Can you work these out from the model? Positions are in its coordinate system, mm. Face numbers are marked on the shaded views. A direction names the side the tool comes from. Give positions to 0.01 mm unless a question says otherwise; leave off trailing zeros. Write each loop counter-clockwise with the first axis right and the second up, starting at its lowest first coordinate (ties: lowest second). Pieces come first, ordered by that corner, then holes.
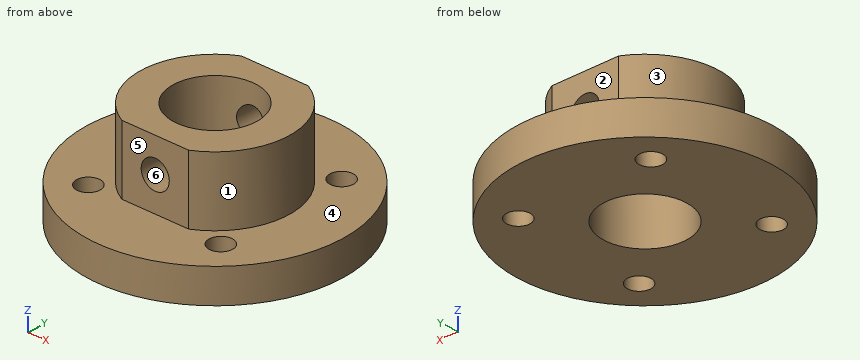
Autodesk Inventor part; units mm, degrees
ref_plane "YZ Plane" through (0, 0, 0) normal (1, 0, 0) x (0, 1, 0)
ref_plane "XZ Plane" through (0, 0, 0) normal (0, 1, 0) x (-1, 0, 0)
ref_plane "XY Plane" through (0, 0, 0) normal (0, 0, 1) x (1, 0, 0)
sketch "スケッチ1" plane through (0, 0, 0) normal (0, 0, 1) x (1, 0, 0)
  circle A0 centre (0, 0) radius 19
  circle A1 centre (0, 0) radius 14
  circle A2 centre (-14, 0) radius 1.75
  circle A3 centre (0, -14) radius 1.75
  circle A4 centre (14, 0) radius 1.75
  circle A5 centre (0, 14) radius 1.75
  line L0 (-19, 0) -> (19, 0)
  dimension "d10" = 28
  dimension "d0" = 38
  dimension "d11" = 3.5
  dimension "d14" = 360
extrude "押し出し1" add sketch "スケッチ1" along normal blind 5
sketch "スケッチ2" plane through (0, 0, 5) normal (0, 0, 1) x (1, 0, 0)
  circle A0 centre (0, 0) radius 11
  line L0 (5, -9.798) -> (-5, -9.798)
  line L1 (-5, -9.798) -> (-5, 9.798)
  line L2 (-5, 9.798) -> (5, 9.798)
  line L3 (5, 9.798) -> (5, -9.798)
  line L4 (5, -9.798) -> (-5, 9.798) construction
  line L5 (-5, -9.798) -> (5, 9.798) construction
  dimension "d3" = 22
  dimension "d6" = 10
extrude "押し出し2" add sketch "スケッチ2" along normal blind 10 contours A0 L3 | L3 L0 L1 L2 | L1 A0
sketch "スケッチ3" plane through (0, 0, 0) normal (0, 0, -1) x (-1, 0, 0)
  circle A0 centre (0, 0) radius 6.2
  dimension "d7" = 12.4
extrude "押し出し3" cut sketch "スケッチ3" against normal blind 30
sketch "スケッチ4" plane through (0, 0, 0) normal (0, 0, -1) x (-1, 0, 0)
  circle A0 centre (0, 0) radius 14
  point P0 (-14, 0)
  point P1 (-9.8995, -9.8995)
  point P2 (0, -14)
  point P3 (9.8995, -9.8995)
  point P4 (14, 0)
  point P5 (9.8995, 9.8995)
  point P6 (0, 14)
  point P7 (-9.8995, 9.8995)
  dimension "d16" = 28
  dimension "d33" = 360
hole "穴1" at (9.8995, -9.8995, 0) at (9.8995, 9.8995, 0) at (-9.8995, 9.8995, 0) at (-9.8995, -9.8995, 0) direction (0, 0, 1) diameter 3.5 end through all
sketch "スケッチ5" plane through (-5, 9.798, 5) normal (0, 1, 0) x (1, 0, 0)
  line L0 (10, -10) -> (0, -10)
  line L1 (5, -10) -> (5, 0)
  line L2 (0, 0) -> (10, 0)
  point P0 (5, 5)
  point P1 (5, -5)
hole "穴2" at (0, 9.798, 10) direction (0, -1, 0) diameter 4.2 end through all
properties part number "light_tire_fixer_10"
(1) Imagine slicing it at B-B, the plane y = 0. Write out the boundary of the cut face in (x, z).
Returned:
outline: (-19, 0) - (-6.2, 0) - (-6.2, 15) - (-11, 15) - (-11, 5) - (-19, 5) - close; (6.2, 0) - (19, 0) - (19, 5) - (11, 5) - (11, 15) - (6.2, 15) - close
(2) If I drill on L1, parallel to Z at x = 0, y = -8; L2, parallel to X at y = 9, z = 3.75; L3, parallel to X at y = 10.5, z = 2.5, over which ranges is the centre line in solid material (lowest first)?
Returned:
L1: z = 0 to 7.9, 12.1 to 15
L2: x = -16.73 to -11.4, -8.4 to 8.4, 11.4 to 16.73
L3: x = -15.84 to -11.54, -8.26 to 8.26, 11.54 to 15.84
(3) Imagine slicing it at D-D, the plane x = 9. Write out the boundary of the cut face in (y, z).
Returned:
outline: (-16.73, 0) - (-11.4, 0) - (-11.4, 5) - (-16.73, 5) - close; (-8.4, 0) - (8.4, 0) - (8.4, 5) - (6.32, 5) - (6.32, 15) - (-6.32, 15) - (-6.32, 5) - (-8.4, 5) - close; (11.4, 0) - (16.73, 0) - (16.73, 5) - (11.4, 5) - close
(4) Will these pins go through, and if not, where does the flat tip stop? P1, Ø4, axis at x = -9.9, y = 9.9, coming from the +Z side; P2, Ø1, axis at y = -2.5, z = 4, coming from the +X side; P3, Ø3, axis at x = 9.9, y = 9.9, coming from the +Z side; P4, Ø1.5, axis at x = 1.5, z = 8.5, coming from the -Y side.
Returned:
P1: stops at z = 5
P2: stops at x = 18.89
P3: passes through
P4: stops at y = -9.8
(5) Imagine slicing it at C-C, the plane z = 10. Write out the boundary of the cut face in (x, y), plus the area to 3 significant figures.
Returned:
outline: (-5, -9.8) - (-2.1, -9.8) - (-2.1, -5.83) arc R6.2 cw to (-2.1, 5.83) - (-2.1, 9.8) - (-5, 9.8) arc R11 ccw to start; (2.1, -9.8) - (5, -9.8) arc R11 ccw to (5, 9.8) - (2.1, 9.8) - (2.1, 5.83) arc R6.2 cw to (2.1, -5.83) - close
area: 212 mm2
(6) Imagine slicing it at A-A, the plane x = 0. Write out the boundary of the cut face in (y, z).
Returned:
outline: (-19, 0) - (-6.2, 0) - (-6.2, 7.9) - (-9.8, 7.9) - (-9.8, 5) - (-19, 5) - close; (-9.8, 12.1) - (-6.2, 12.1) - (-6.2, 15) - (-9.8, 15) - close; (6.2, 0) - (19, 0) - (19, 5) - (9.8, 5) - (9.8, 7.9) - (6.2, 7.9) - close; (6.2, 12.1) - (9.8, 12.1) - (9.8, 15) - (6.2, 15) - close
(7) For the marked faces 1, 2 and 3, which set-ups out of +Z, -Z, +X, -X, +Y, -Y let a thin tool reach every point of the face, with its end or its side?
Returned:
face 1: +Z, +X
face 2: +Z, +X, -X, +Y
face 3: +Z, -X
(8) If we mould it in two halves opening along Z, with no side actions, what happens to the marked faces 4, 5 and 6? For each: +Z half, -Z half, draft (parallel to the pull), parting line (faces both ways), or undercut.
Returned:
face 4: +Z half
face 5: draft
face 6: undercut
